Work out the finished part from the listing and answer in its coordinate system (mm). Round coordinates to 2 decimals unless told otherwise and drop trailing zeros. Write each loop counter-clockwise with the first axis right and the second up, starting at its lowest first coordinate (ties: lowest second). Pieces come first, ordered by that corner, then holes. Notation, with made-up numbers: M 27.5,-35 L 41.5,-35 A30 cw 41.5,1 Z; hole C 36.5,80 d4. An arc over 180 degrees is marked long. Answer in a Markdown table with one row per item.
```python
from build123d import *

# Parameters (mm, degrees)
SKETCH1_W                   = 228.6
SKETCH1_H                   = 349.25
SKETCH1_W_2                 = 101.6
SKETCH1_H_2                 = 121.92
BOSS_EXTRUDE1_DEPTH         = 2.667
CORNERRADIUSALLOWANCE_DEPTH = 368.487639777


with BuildPart() as part:
    # Sketch1 → Boss-Extrude1 (new body)
    with BuildSketch(Plane(origin=(0, 0, 0), x_dir=(0, 0, -1), z_dir=(1, 0, 0))):
        with Locations((0, 174.625)):
            Rectangle(SKETCH1_W, SKETCH1_H)
        with BuildLine():
            Line((98.1075, 207.645), (58.7375, 207.645))
            ThreePointArc((58.7375, 207.645), (56.49243597, 208.57493597), (55.5625, 210.82))
            Line((55.5625, 210.82), (55.5625, 318.77))
            ThreePointArc((55.5625, 318.77), (56.49243597, 321.01506403), (58.7375, 321.945))
            Line((58.7375, 321.945), (98.1075, 321.945))
            ThreePointArc((98.1075, 321.945), (100.35256403, 321.01506403), (101.2825, 318.77))
            Line((101.2825, 318.77), (101.2825, 210.82))
            ThreePointArc((101.2825, 210.82), (100.35256403, 208.57493597), (98.1075, 207.645))
        make_face(mode=Mode.SUBTRACT)
        with Locations((0, 264.795)):
            Rectangle(SKETCH1_W_2, SKETCH1_H_2, mode=Mode.SUBTRACT)
        with BuildLine():
            Line((-98.1075, 207.645), (-58.7375, 207.645))
            ThreePointArc((-58.7375, 207.645), (-56.49243597, 208.57493597), (-55.5625, 210.82))
            Line((-55.5625, 210.82), (-55.5625, 318.77))
            ThreePointArc((-55.5625, 318.77), (-56.49243597, 321.01506403), (-58.7375, 321.945))
            Line((-58.7375, 321.945), (-98.1075, 321.945))
            ThreePointArc((-98.1075, 321.945), (-100.35256403, 321.01506403), (-101.2825, 318.77))
            Line((-101.2825, 318.77), (-101.2825, 210.82))
            ThreePointArc((-101.2825, 210.82), (-100.35256403, 208.57493597), (-98.1075, 207.645))
        make_face(mode=Mode.SUBTRACT)
    extrude(amount=BOSS_EXTRUDE1_DEPTH)

    # Sketch2 → CornerRadiusAllowance (cut, through all)
    with BuildSketch(Plane(origin=(2.667, 0, 0), x_dir=(0, 0, -1), z_dir=(1, 0, 0))):
        Polygon((114.3, 349.25), (-114.3, 349.25), (-114.3, 0), (-107.95, 0), (-107.95, 342.9), (107.95, 342.9), (107.95, 0), (114.3, 0), align=None)
    extrude(amount=-CORNERRADIUSALLOWANCE_DEPTH, mode=Mode.SUBTRACT)


solid = part.part
```
1. The part is cut by section C-C (z = 35). Determine the outline of the cut face in (x, y) (3 decimals), plus the area to 3 significant figures.
Calculated:
| item | result |
|---|---|
| outline | M 0,0 L 2.667,0 L 2.667,203.835 L 0,203.835 Z; M 0,325.755 L 2.667,325.755 L 2.667,342.9 L 0,342.9 Z |
| area | 589 mm² |
2. The part is cut by section A-A (y = 284). Determine the outline of the cut face in (x, z), plus the area to 3 significant figures.
Calculated:
| item | result |
|---|---|
| outline | M 0,-107.95 L 2.67,-107.95 L 2.67,-101.28 L 0,-101.28 Z; M 0,-55.56 L 2.67,-55.56 L 2.67,-50.8 L 0,-50.8 Z; M 0,50.8 L 2.67,50.8 L 2.67,55.56 L 0,55.56 Z; M 0,101.28 L 2.67,101.28 L 2.67,107.95 L 0,107.95 Z |
| area | 61.0 mm² |
3. Consider line 1 along Z through (x, y) = (1.1, 266); line 2 along Y through (x, z) = (0.75, 61.5) (3 decimals); line 3 along Y through (x, z) = (1.5, 0) (3 decimals). Determine where each line is inside the solid, lowest interval first. Write a range as from..to.
Calculated:
| item | result |
|---|---|
| line 1 | z = -107.95..-101.28, -55.56..-50.8, 50.8..55.56, 101.28..107.95 |
| line 2 | y = 0..207.645, 321.945..342.9 |
| line 3 | y = 0..203.835, 325.755..342.9 |
4. The part is cut by section B-B (x = 1). Count the separate pieces of the cut face and the enclosed holes in it, plus the area to 3 significant figures.
Calculated:
| item | result |
|---|---|
| separate pieces | 1 |
| enclosed holes | 3 |
| area | 51,200 mm² |
5. Given pin 1 (2 mm diameter, centred on y = 216, z = 55, fed in from -X), flat-ended and moving along its own axis, determine where the tip first touches the part or whether it passes through.
Calculated:
| item | result |
|---|---|
| pin 1 | stops at x = 0 |
